```python
from build123d import *

# Parameters (mm, degrees)
PAD012_DEPTH    = 10
SKETCH027_W     = 3.4
SKETCH027_H     = 5
POCKET_DEPTH    = 30
POCKET012_DEPTH = 247.759716
SKETCH029_R     = 11
POCKET013_DEPTH = 3.5
POCKET014_DEPTH = 5
SKETCH031_R     = 2.2
POCKET015_DEPTH = 5.001
POCKET016_DEPTH = 243.669334
FILLET_R        = 0.5
FILLET001_R     = 1
FILLET002_R     = 1
SKETCH048_R     = 3.75
PAD019_DEPTH    = 5
SKETCH049_R     = 4.693549
POCKET026_DEPTH = 2.5
FILLET012_R     = 0.5
PAD020_DEPTH    = 5
FILLET013_R     = 1
PAD021_DEPTH    = 7.5
POCKET029_DEPTH = 5
POCKET030_DEPTH = 18
SKETCH055_W     = 3.4
SKETCH055_H     = 44.110421
POCKET031_DEPTH = 10
POCKET032_DEPTH = 3.5
SKETCH057_R     = 3.2
POCKET033_DEPTH = 3.5
FILLET018_R     = 4
FILLET019_R     = 1


with BuildPart() as part:
    # Sketch026 (on ShapeBinder) → Pad012 (new body)
    with BuildSketch(Plane.XZ.offset(47.5)):
        with BuildLine():
            ThreePointArc((18, -27.658633), (33, 0), (18, 27.658633))
            Line((18, 27.658633), (9, 27.658633))
            Line((9, 31.749016), (9, 27.658633))
            Line((-9, 31.749016), (9, 31.749016))
            Line((-9, 31.749016), (-9, 27.658633))
            Line((-18, 27.658633), (-9, 27.658633))
            ThreePointArc((-18, 27.658633), (-33, 0), (-18, -27.658633))
            Line((-18, -27.658633), (-9, -27.658633))
            Line((-9, -31.749016), (-9, -27.658633))
            Line((-9, -31.749016), (9, -31.749016))
            Line((9, -31.749016), (9, -27.658633))
            Line((18, -27.658633), (9, -27.658633))
        make_face()
        with BuildLine():
            ThreePointArc((-1.45, -12.6), (0, -14.05), (1.45, -12.6))
            Line((1.45, -12.6), (1.45, -11.15))
            ThreePointArc((1.45, -11.15), (0, -9.7), (-1.45, -11.15))
            Line((-1.45, -12.6), (-1.45, -11.15))
        make_face(mode=Mode.SUBTRACT)
    extrude(amount=PAD012_DEPTH)

    # Sketch027 (on Face4 of Pad012) → Pocket (cut)
    with BuildSketch(Plane(origin=(0, -4.5, 31.749016), x_dir=(1, 0, 0), z_dir=(0, 0, 1))):
        with Locations((0, -45.5)):
            Rectangle(SKETCH027_W, SKETCH027_H)
    extrude(amount=-POCKET_DEPTH, mode=Mode.SUBTRACT)

    # Sketch028 (on Face14 of Pocket) → Pocket012 (cut, through all)
    with BuildSketch(Plane(origin=(0, -4.5, 31.749016), x_dir=(1, 0, 0), z_dir=(0, 0, 1))):
        with BuildLine():
            Line((-6.074874, -48.75), (-4.625126, -48.75))
            Line((-4.112563, -49.262563), (-4.625126, -48.75))
            ThreePointArc((-6.587437, -49.262563), (-5.35, -52.25), (-4.112563, -49.262563))
            Line((-6.074874, -48.75), (-6.587437, -49.262563))
        make_face()
        with BuildLine():
            Line((4.625126, -48.75), (6.074874, -48.75))
            Line((6.587437, -49.262563), (6.074874, -48.75))
            ThreePointArc((4.112563, -49.262563), (5.35, -52.25), (6.587437, -49.262563))
            Line((4.625126, -48.75), (4.112563, -49.262563))
        make_face()
    extrude(amount=-POCKET012_DEPTH, mode=Mode.SUBTRACT)

    # Sketch029 (on Face4 of Pocket012) → Pocket013 (cut)
    with BuildSketch(Plane(origin=(0, -47.5, 0), x_dir=(-1, 0, 0), z_dir=(0, 1, 0))):
        with Locations((0, -12.6)):
            Circle(SKETCH029_R)
    extrude(amount=-POCKET013_DEPTH, mode=Mode.SUBTRACT)

    # Sketch030 (on Face5 of Pocket013) → Pocket014 (cut)
    with BuildSketch(Plane.XZ.offset(57.5)):
        Polygon((27.036196, -16.3), (29.172392, -12.6), (27.036196, -8.9), (22.763804, -8.9), (20.627608, -12.6), (22.763804, -16.3), align=None)
        Polygon((-22.763804, -16.3), (-20.627608, -12.6), (-22.763804, -8.9), (-27.036196, -8.9), (-29.172392, -12.6), (-27.036196, -16.3), align=None)
    extrude(amount=-POCKET014_DEPTH, mode=Mode.SUBTRACT)

    # Sketch031 (on Face46 of Pocket014) → Pocket015 (cut, through all)
    with BuildSketch(Plane.XZ.offset(52.5)):
        with Locations((24.9, -12.6)):
            Circle(SKETCH031_R)
        with Locations((-24.9, -12.6)):
            Circle(SKETCH031_R)
    extrude(amount=-POCKET015_DEPTH, mode=Mode.SUBTRACT)

    # Sketch032 (on Face3 of Pocket015) → Pocket016 (cut, through all)
    with BuildSketch(Plane(origin=(0, -4.5, 27.658633), x_dir=(1, 0, 0), z_dir=(0, 0, 1))):
        with BuildLine():
            Line((11.025126, -48.75), (12.474874, -48.75))
            Line((12.474874, -48.75), (12.987437, -49.262563))
            ThreePointArc((10.512563, -49.262563), (11.75, -52.25), (12.987437, -49.262563))
            Line((11.025126, -48.75), (10.512563, -49.262563))
        make_face()
        with BuildLine():
            Line((15.025126, -44.125), (16.474874, -44.125))
            Line((16.474874, -44.125), (16.987437, -44.637563))
            ThreePointArc((14.512563, -44.637563), (15.75, -47.625), (16.987437, -44.637563))
            Line((15.025126, -44.125), (14.512563, -44.637563))
        make_face()
    pocket016 = extrude(amount=-POCKET016_DEPTH, mode=Mode.SUBTRACT)

    # Mirrored: Pocket016 across Sketch032 V_Axis
    add(pocket016.mirror(Plane(origin=(0, -4.5, 27.658633), x_dir=(0, 0, 1), z_dir=(1, 0, 0))), mode=Mode.SUBTRACT)

    # Fillet
    fillet_edges = [part.edges().sort_by_distance(p)[0] for p in [
        (-1.7, -52.5, 16.749016),
        (1.7, -52.5, 16.749016),
    ]]
    fillet(fillet_edges, radius=FILLET_R)

    # Fillet001
    fillet001_edges = [part.edges().sort_by_distance(p)[0] for p in [
        (-9, -52.5, 31.749016),
        (9, -52.5, 31.749016),
    ]]
    fillet(fillet001_edges, radius=FILLET001_R)

    # Fillet002
    fillet002_edges = [part.edges().sort_by_distance(p)[0] for p in [
        (9, -52.5, -31.749016),
        (-9, -52.5, -31.749016),
    ]]
    fillet(fillet002_edges, radius=FILLET002_R)

    # Sketch048 (on Face53 of Fillet002) → Pad019 (join)
    with BuildSketch(Plane(origin=(0, -51, 0), x_dir=(-1, 0, 0), z_dir=(0, 1, 0))):
        with Locations((0, -12.6)):
            Circle(SKETCH048_R)
        with BuildLine():
            ThreePointArc((1.45, -11.15), (0, -9.7), (-1.45, -11.15))
            Line((-1.45, -11.15), (-1.45, -12.6))
            ThreePointArc((-1.45, -12.6), (0, -14.05), (1.45, -12.6))
            Line((1.45, -11.15), (1.45, -12.6))
        make_face(mode=Mode.SUBTRACT)
    extrude(amount=PAD019_DEPTH)

    # Sketch049 (on Face24 of Pad019) → Pocket026 (cut)
    with BuildSketch(Plane.XZ.offset(57.5)):
        with Locations((-24.9, -12.6)):
            Circle(SKETCH049_R)
        with Locations((24.9, -12.6)):
            Circle(SKETCH049_R)
    extrude(amount=-POCKET026_DEPTH, mode=Mode.SUBTRACT)

    # Fillet012
    fillet012_edges = [part.edges().sort_by_distance(p)[0] for p in [
        (3.75, -51, -12.6),
    ]]
    fillet(fillet012_edges, radius=FILLET012_R)

    # Sketch050 (on Face76 of Pad019) → Pad020 (join)
    with BuildSketch(Plane(origin=(0, -46, 0), x_dir=(-1, 0, 0), z_dir=(0, 1, 0))):
        with BuildLine():
            ThreePointArc((-1.45, -9.141677), (0, -16.35), (1.45, -9.141677))
            Line((1.45, -12.6), (1.45, -9.141677))
            ThreePointArc((-1.45, -12.6), (0, -14.05), (1.45, -12.6))
            Line((-1.45, -12.6), (-1.45, -9.141677))
        make_face()
    extrude(amount=PAD020_DEPTH)

    # Fillet013
    fillet013_edges = [part.edges().sort_by_distance(p)[0] for p in [
        (0, -41, -16.35),
    ]]
    fillet(fillet013_edges, radius=FILLET013_R)

    # Sketch053 (on Face39 of Fillet013) → Pad021 (join)
    with BuildSketch(Plane(origin=(0, -47.5, 0), x_dir=(-1, 0, 0), z_dir=(0, 1, 0))):
        with BuildLine():
            Line((-8, 31.749016), (8, 31.749016))
            ThreePointArc((9, 30.749016), (8.707107, 31.456123), (8, 31.749016))
            Line((9, 30.749016), (9, 19.658633))
            Line((9, 19.658633), (-9, 19.658633))
            Line((-9, 19.658633), (-9, 30.749016))
            ThreePointArc((-8, 31.749016), (-8.707107, 31.456123), (-9, 30.749016))
        make_face()
    extrude(amount=PAD021_DEPTH)

    # Sketch030 (on Face5 of Pocket013) → Pocket029 (cut)
    with BuildSketch(Plane.XZ.offset(57.5)):
        Polygon((27.036196, -16.3), (29.172392, -12.6), (27.036196, -8.9), (22.763804, -8.9), (20.627608, -12.6), (22.763804, -16.3), align=None)
        Polygon((-22.763804, -16.3), (-20.627608, -12.6), (-22.763804, -8.9), (-27.036196, -8.9), (-29.172392, -12.6), (-27.036196, -16.3), align=None)
    extrude(amount=-POCKET029_DEPTH, mode=Mode.SUBTRACT)

    # Sketch054 (on Face56 of Pocket029) → Pocket030 (cut)
    with BuildSketch(Plane(origin=(9, -4.5, 0), x_dir=(0, 1, 0), z_dir=(1, 0, 0))):
        with BuildLine():
            ThreePointArc((-38.012563, 26.441261), (-41, 25.203825), (-38.012563, 23.966388))
            Line((-38.012563, 23.966388), (-37.5, 24.478951))
            Line((-37.5, 25.928698), (-37.5, 24.478951))
            Line((-37.5, 25.928698), (-38.012563, 26.441261))
        make_face()
    extrude(amount=-POCKET030_DEPTH, mode=Mode.SUBTRACT)

    # Sketch055 (on Face39 of Pocket030) → Pocket031 (cut)
    with BuildSketch(Plane(origin=(0, -47.5, 0), x_dir=(-1, 0, 0), z_dir=(0, 1, 0))):
        with Locations((0, 23.804226)):
            Rectangle(SKETCH055_W, SKETCH055_H)
    extrude(amount=POCKET031_DEPTH, mode=Mode.SUBTRACT)

    # Sketch056 (on Face56 of Pocket031) → Pocket032 (cut)
    with BuildSketch(Plane(origin=(9, -4.5, 0), x_dir=(0, 1, 0), z_dir=(1, 0, 0))):
        Polygon((-36.35, 23.529509), (-36.35, 26.87814), (-39.25, 28.552456), (-42.15, 26.87814), (-42.15, 23.529509), (-39.25, 21.855193), align=None)
    extrude(amount=-POCKET032_DEPTH, mode=Mode.SUBTRACT)

    # Sketch057 (on Face74 of Pocket032) → Pocket033 (cut)
    with BuildSketch(Plane(origin=(-9, -4.5, 0), x_dir=(0, -1, 0), z_dir=(-1, 0, 0))):
        with Locations((39.25, 25.203825)):
            Circle(SKETCH057_R)
    extrude(amount=-POCKET033_DEPTH, mode=Mode.SUBTRACT)

    # Fillet018
    fillet018_edges = [part.edges().sort_by_distance(p)[0] for p in [
        (-5.35, -47.5, 19.658633),
        (5.35, -47.5, 19.658633),
    ]]
    fillet(fillet018_edges, radius=FILLET018_R)

    # Fillet019
    fillet019_edges = [part.edges().sort_by_distance(p)[0] for p in [
        (5.35, -40, 19.658633),
        (-5.35, -40, 19.658633),
    ]]
    fillet(fillet019_edges, radius=FILLET019_R)


solid = part.part
```
Design review of the part built by this model. Coordinates are the model's own, in mm. A direction names the side the tool comes from. Give positions to 0.01 mm unless a question says otherwise; leave off trailing zeros. Write each loop counter-clockwise with the first axis right and the second up, starting at its lowest first coordinate (ties: lowest second). Pieces come first, ordered by that corner, then holes. Notation, with made-up numbers: (15, 43.25) - (36, 43.25) arc R31 cw to (36, 78.25) - close; hole circle Ø7 at (14, -21). An arc over 180 degrees is marked (long way). Return JSON: item names as keys, results as strings. Group by question number.
(1) We need section D-D, the plane x = -24. Give the boundary of the cut face in (y, z), then the cut area to 3 significant figures.
(2) Machinability: for faces 4 (the flat face through (-16, -48.625, 0)), 5 (the cylindrical face through (-5.299, -46.359, 18.456)), 6 (the flat face through (-25, -54, -8.9)), 7 (the flat face through (-1.7, -47, 20)), which of the approach directions +Z, -Z, +X, -X, +Y, -Y give a long, thin tool a straight path to every point of the face, cutting with its end or side? Answer none if there is none.
(3) We need section B-B, the plane z = 9. Give the number of separate pieces and of enclosed holes in the cut face, then the cut area to 3 significant figures.
(4) We need section A-A, the plane x = 0. Give the boundary of the cut face in (y, z).
(5) To check wall thickness, follow probe 1 along Z at (x, y) = (0, -49); probe 2 along Z at (x, y) = (2.85, -43.75); probe 3 along X at (y, z) = (-48.75, 1.5). State the ranges of each line that lie inside material, in increasing order.
(6) Mouldability with a two-part tool opening along Y and no side actions: class faces 1 (the flat face through (14, -52, 27.659)), 2 (the flat face through (5, -53.25, 0)), 3 (the flat face through (-28, -55, -10)) as +Y half, -Y half, draft (parallel to the pull), parting line (faces both ways), or undercut.
(7) Insertion check: pin 1 (2 mm diameter, centred on x = -21, y = -47.5, fed in from +Z); pin 2 (10 mm diameter, centred on x = -12.5, y = -42, fed in from -Z); pin 3 (18 mm diameter, centred on x = 15.5, z = -9.5, fed in from +Y). Each pin has a flat end and moves straight along its axis. Give the tip position at first contact, or say it passes through.
Reported:
{
 "1": {"outline": "(-57.5, -22.65) - (-47.5, -22.65) - (-47.5, -14.61) - (-52.5, -14.61) - (-52.5, -16.3) - (-55, -16.3) - (-55, -17.21) - (-57.5, -17.21) - close; (-57.5, -7.99) - (-55, -7.99) - (-55, -8.9) - (-52.5, -8.9) - (-52.5, -10.59) - (-47.5, -10.59) - (-47.5, 22.65) - (-57.5, 22.65) - close", "area": "391 mm2"},
 "2": {"face 4": "+Z, -Z", "face 5": "+X, -X, +Y", "face 6": "-Y", "face 7": "+Z, +Y"},
 "3": {"separate pieces": "1", "enclosed holes": "6", "area": "560 mm2"},
 "4": {"outline": "(-57.5, -31.75) - (-47.5, -31.75) - (-47.5, -23.6) - (-51, -23.6) - (-51, -16.85) arc R0.5 cw to (-50.5, -16.35) - (-42, -16.35) arc R1 ccw to (-41, -15.35) - (-41, -14.05) - (-57.5, -14.05) - close; (-57.5, -9.7) - (-46, -9.7) - (-46, -8.85) - (-50.5, -8.85) arc R0.5 cw to (-51, -8.35) - (-51, -1.6) - (-47.5, -1.6) - (-47.5, 1.75) - (-52.5, 1.75) - (-52.5, 31.75) - (-57.5, 31.75) - close"},
 "5": {"probe 1": "z = -31.75 to -23.6, -16.35 to -14.05, -9.7 to -8.85, -1.6 to 1.75", "probe 2": "z = -15.04 to -10.16, 19.65 to 23.45, 26.95 to 31.75", "probe 3": "x = -32.97 to -16.6, -14.9 to 14.9, 16.6 to 32.97"},
 "6": {"face 1": "draft", "face 2": "undercut", "face 3": "-Y half"},
 "7": {"pin 1": "stops at z = 26.25", "pin 2": "stops at z = 19.08", "pin 3": "stops at y = -47.5"}
}
